Geometry check sheet. Reference: drawing and pictorial views, mm from the part's lowest x, y, z. Coordinates: 2 decimals unless noted, no trailing zeros. Write each loop counter-clockwise with the first axis right and the second up, starting at its lowest first coordinate (ties: lowest second). Pieces come first, ordered by that corner, then holes. Notation, with made-up numbers: (28, -10.5) - (38, -10.5) arc R26 ccw to (38, 5.5) - close; hole circle Ø7 at (87.25, 49). An arc over 180 degrees is marked (long way). Use one line per item in the form item = value. Start each with the question number.
(1) Sectioned sample at C-C (y = 10.75). Record the cut outline in (x, z), and give its area (3 significant figures).
(2) Material ranges on line 1 (Z direction, x = 110, y = 1.75); line 2 (X direction, y = 2, z = 70.5); line 3 (Z direction, x = 198.5, y = 15.5) (1 decimal), recorded low to high. Write a range as [from, to].
(3) Gauge pin test, flat ends, axial feed: pin 1 Ø2 at (y, z) = (21, 341) entering from +X; pin 2 Ø5 at (x, y) = (44, 19) entering from -Z (1 decimal); pin 3 Ø5 at (x, y) = (299.5, 20) entering from -Z. Record the tip position at first contact, or that the pin passes through.
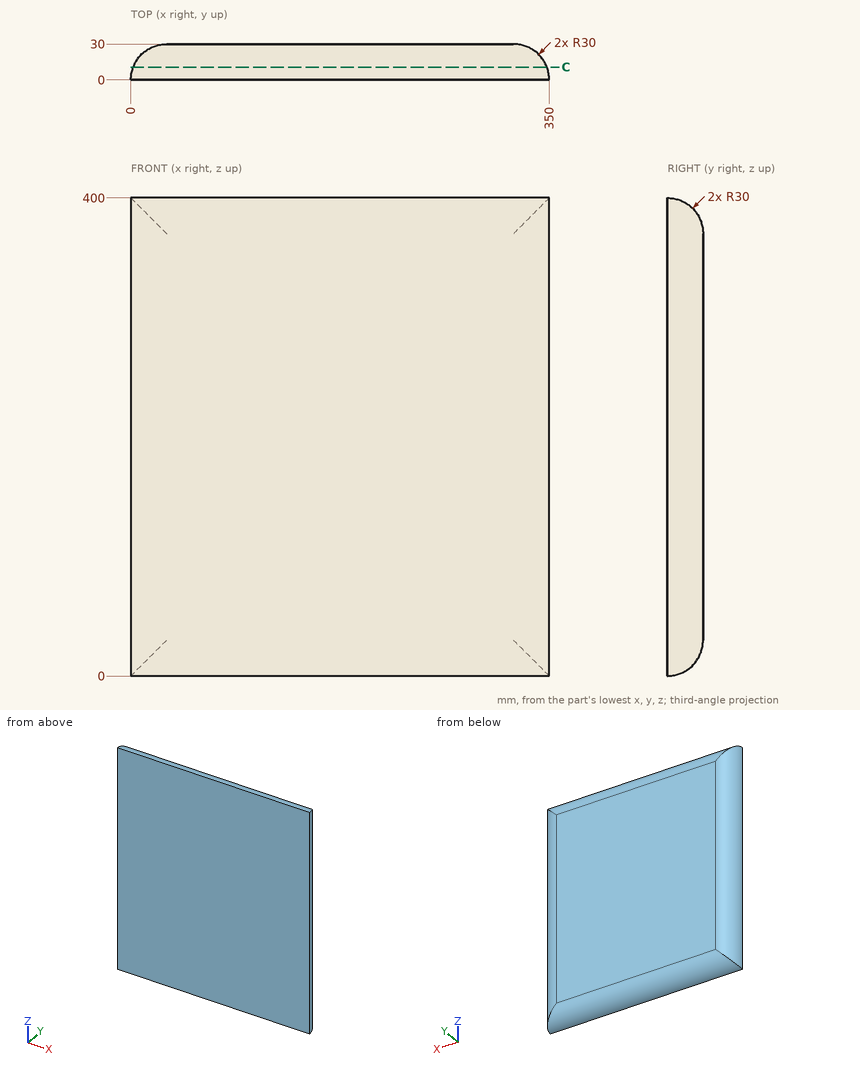
Answers below:
q1.outline = (1.99, 1.99) - (348.01, 1.99) - (348.01, 398.01) - (1.99, 398.01) - close
q1.area = 137,000 mm2
q2.line_1 = [0.05, 399.95]
q2.line_2 = [0.07, 349.93]
q2.line_3 = [4.3, 395.7]
q3.pin_1 = 342.36
q3.pin_2 = 4.9
q3.pin_3 = 5.63
